from build123d import *

# Parameters (mm, degrees)
SKETCH2_R           = 10
CUT_EXTRUDE2_DEPTH  = 20
SKETCH3_R           = 7.5
SKETCH3_R_2         = 6.5
BOSS_EXTRUDE2_DEPTH = 1.5


with BuildPart() as part:
    # Sketch1 → Revolve1 (revolve)
    with BuildSketch(Plane.XY, mode=Mode.PRIVATE) as revolve1_sk:
        Polygon((0, 140), (-15, 140), (-15, 115), (-6, 106), (-6, 30), (-60, 10), (-60, 0), (0, 0), align=None)
    revolve(revolve1_sk.sketch.rotate(Axis((0, 0, 0), (0, 1, 0)), 270), axis=Axis((0, 0, 0), (0, 1, 0)))

    # Sketch2 → Cut-Extrude2 (cut)
    with BuildSketch(Plane(origin=(0, 140, 0), x_dir=(1, 0, 0), z_dir=(0, 1, 0))):
        with Locations(Location((0, 0, 0), (0, 0, 270))):
            Circle(SKETCH2_R)
    extrude(amount=-CUT_EXTRUDE2_DEPTH, mode=Mode.SUBTRACT)

    # Sketch3 → Boss-Extrude2 (add, symmetric)
    with BuildSketch(Plane.XY):
        with Locations((31, 26.072659277)):
            Circle(SKETCH3_R)
        with Locations((31, 26.072659277)):
            Circle(SKETCH3_R_2, mode=Mode.SUBTRACT)
    extrude(amount=BOSS_EXTRUDE2_DEPTH, both=True)


solid = part.part
Geometry check sheet. Reference: the model listing, model coordinates, mm. A direction names the side the tool comes from. Round coordinates to 2 decimals unless told otherwise and drop trailing zeros. Write each loop counter-clockwise with the first axis right and the second up, starting at its lowest first coordinate (ties: lowest second). Pieces come first, ordered by that corner, then holes.
Item 1: Go/stop test with flat-tipped pins: pin 1 Ø4 at (x, z) = (-46, 27) entering from +Y; pin 2 Ø1.5 at (x, z) = (-5.5, -39.5) entering from +Y; pin 3 Ø10 at (x, z) = (4.5, 1) entering from +Y; pin 4 Ø4 at (x, y) = (32.5, 23.5) entering from -Z. Record where each tip stops, or that it passes through.
Determined:
pin 1: stops at y = 13.21
pin 2: stops at y = 17.73
pin 3: stops at y = 120
pin 4: passes through
Item 2: Material ranges on line 1 along X through (y, z) = (124.5, 0); line 2 along Y through (x, z) = (31, 0.85); line 3 along X through (y, z) = (123.5, 7), recorded low to high.
Determined:
line 1: x = -15 to -10, 10 to 15
line 2: y = 0 to 20.74, 32.57 to 33.57
line 3: x = -13.27 to -7.14, 7.14 to 13.27
Item 3: Section check C-C (y = 16.5). Record the boundary of the cut face in (x, z).
Determined:
outline: circle Ø84.9 at (0, 0)
Item 4: Section check B-B (y = 43.5). Record the boundary of the cut face in (x, z), plus the area to 3 significant figures.
Determined:
outline: circle Ø12 at (0, 0)
area: 113 mm2
Item 5: Access from +Z, -Z, +X, -X, +Y, -Y to the whole of each face (thin tool, end or side, straight path). Record for faces 1 (the face through (32, 33, -1.5)), 2 (the face through (0, 120, 0)), 3 (the face through (-1.802, 67.468, -5.723)), 4 (the face through (32, 33, 1.5)).
Determined:
face 1: -Z, +X, +Y
face 2: +Y
face 3: none
face 4: +Z, +X, +Y
Item 6: Section check A-A (x = 0). Record the boundary of the cut face in (y, z).
Determined:
outline: (0, -60) - (10, -60) - (30, -6) - (106, -6) - (115, -15) - (140, -15) - (140, -10) - (120, -10) - (120, 10) - (140, 10) - (140, 15) - (115, 15) - (106, 6) - (30, 6) - (10, 60) - (0, 60) - close
Item 7: Mould release check, pull along X, two halves, no side actions. Record for faces 5 (the face through (-9.76, 130.14, -2.17)), 6 (the face through (-1, 0, 1)), 7 (the face through (-0.66, 127.325, 14.985)): +X half, -X half, draft (parallel to the pull), parting line (faces both ways), or undercut.
Determined:
face 5: undercut
face 6: draft
face 7: parting line
